Autodesk Fusion 360 part; units mm, degrees
sketch "Sketch1" plane through (0, 0, 0) normal (0, 1, 0) x (1, 0, 0)
  circle A0 centre (0, 0) radius 1.5
  dimension "d1" = 3
extrude "Extrude1" add sketch "Sketch1" along normal blind 500
extrude "Extrude2" add 1 faces at (0.567, 500, 0.5383) along direction (0, 1, 0) blind 5
extrude "Extrude3" add 1 faces at (0.567, 505, 0.5383) along direction (0, 1, 0) blind 4
Could you check a few things on this model? Use its own coordinates, in mm. Give positions to 0.01 mm unless a question says otherwise; leave off trailing zeros. Write each loop counter-clockwise with the first axis right and the second up, starting at its lowest first coordinate (ties: lowest second). Pieces come first, ordered by that corner, then holes. Notation, with made-up numbers: (-17, 23.5) - (-9, 23.5) arc R19 cw to (-9, 33.5) - close; hole circle Ø9 at (41.5, 78.25). An arc over 180 degrees is marked (long way). One line per item, written item: value. Start each with the question number.
Item 1: Imagine slicing it at B-B, the plane z = 0.9. List the corners of the cut face in (x, y) for me.
Item 2: Imagine slicing it at A-A, the plane y = 166.5. List the corners of the cut face in (x, z) for me.
Item 3: Imagine slicing it at C-C, the plane x = -0.8. List the corners of the cut face in (y, z) for me.
Item 4: Please list where these lines run through material, in increasing order: line 1 (Z direction, x = 0.1, y = 380.5); line 2 (X direction, y = 316.5, z = 0.7); line 3 (Z direction, x = 0.65, y = 303.5). Write a range as from..to.
Geometry says:
1. outline: (-1.2, 0) - (1.2, 0) - (1.2, 509) - (-1.2, 509) - close
2. outline: circle Ø3 at (0, 0)
3. outline: (0, -1.27) - (509, -1.27) - (509, 1.27) - (0, 1.27) - close
4. line 1: -1.5..1.5
4. line 2: -1.33..1.33
4. line 3: -1.35..1.35
